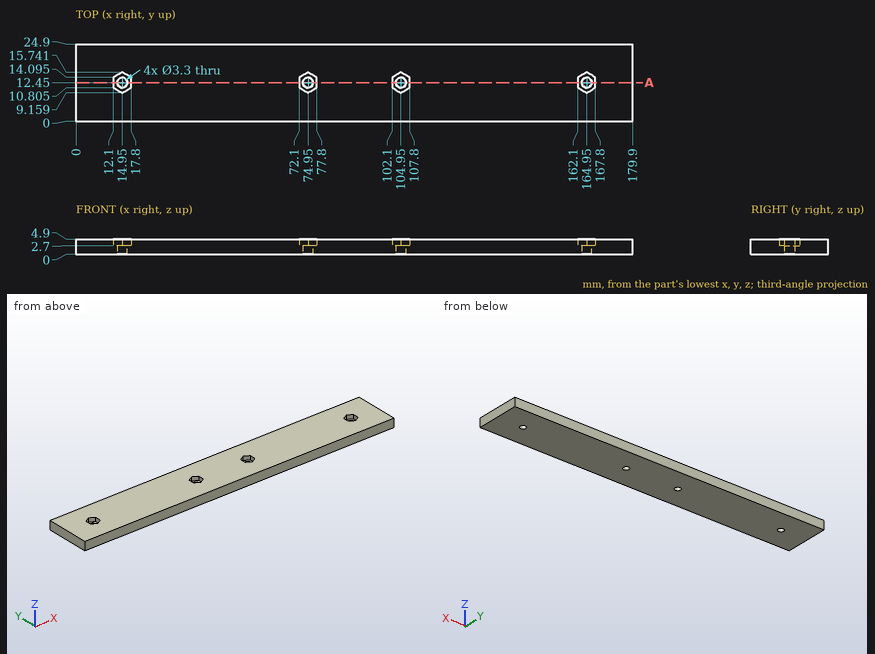
Source: three-view drawing plus pictorial views. Frame: mm from the lowest corner of the part. Coordinates: 2 decimals unless noted, no trailing zeros. Answer as a JSON object with one key per item and string values.
1. Material intervals for line 1 (X direction, y = 12.45, z = 1.4); line 2 (Y direction, x = 164.95, z = 1.8); line 3 (X direction, y = 12, z = 2.45), sorted ascending. Write a range as from..to.
Result set:
{"line 1": "x = 0..13.3, 16.6..73.3, 76.6..103.3, 106.6..163.3, 166.6..179.9", "line 2": "y = 0..10.8, 14.1..24.9", "line 3": "x = 0..13.36, 16.54..73.36, 76.54..103.36, 106.54..163.36, 166.54..179.9"}
2. Section A-A on y = 12.45. Count the separate pieces of the cut face and the enclosed holes in it.
Result set:
{"separate pieces": "5", "enclosed holes": "0"}
3. First-contact query: P1, Ø5.5, axis at x = 74.95, y = 12.45, coming from the +Z side. Flat tip, straight axial feed; report the tip coordinate or a pass-through.
Result set:
{"P1": "stops at z = 2.7"}
